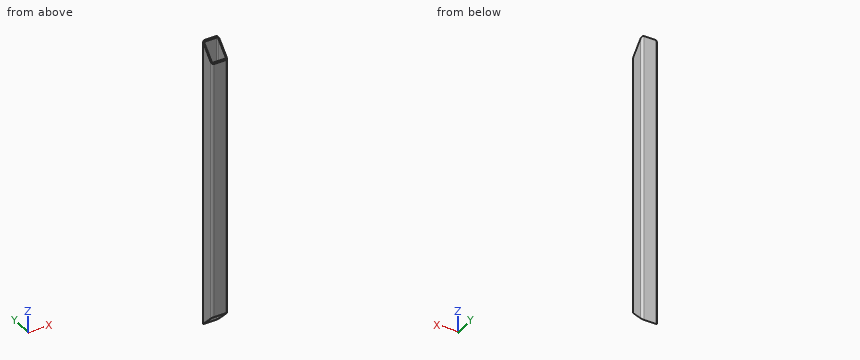
Autodesk Inventor part; units mm, degrees
ref_plane "Plano inicial" through (0, 0, 0) normal (0, 0, 1) x (1, 0, 0)
ref_plane "Plano final" through (0, 0, 550) normal (0, 0, 1) x (1, 0, 0)
ref_plane "Plano de trabalho6" through (15, 0, 0) normal (0, 0, -1) x (-1, 0, 0)
ref_plane "Plano inicial" through (0, 0, 0) normal (0, 0, 1) x (1, 0, 0)
ref_plane "Plano final" through (0, 0, 550) normal (0, 0, 1) x (1, 0, 0)
sketch "Esboço" plane through (0, 0, 0) normal (0, 0, 1) x (1, 0, 0)
  line L0 (-15, -11) -> (-15, 11)
  line L1 (-11, 15) -> (11, 15)
  line L2 (15, 11) -> (15, -11)
  line L3 (11, -15) -> (-11, -15)
  arc A0 (-15, -11) -> (-11, -15) centre (-11, -11) ccw
  arc A1 (15, 11) -> (11, 15) centre (11, 11) ccw
  arc A2 (-11, 15) -> (-15, 11) centre (-11, 11) ccw
  arc A3 (11, -15) -> (15, -11) centre (11, -11) ccw
  arc A4 (-11, 13) -> (-13, 11) centre (-11, 11) ccw
  line L4 (-11, 13) -> (11, 13)
  arc A5 (13, 11) -> (11, 13) centre (11, 11) ccw
  line L5 (13, 11) -> (13, -11)
  arc A6 (11, -13) -> (13, -11) centre (11, -11) ccw
  line L6 (11, -13) -> (-11, -13)
  arc A7 (-13, -11) -> (-11, -13) centre (-11, -11) ccw
  line L7 (-13, -11) -> (-13, 11)
  line L8 (0, 22.1598) -> (0, -22.1598) construction
  line L9 (-22.1598, 0) -> (22.1598, 0) construction
  dimension "d7" = 4
  dimension "d9" = 30
  dimension "d11" = 30
  dimension "d12" = 2
  dimension "d15" = 15
  dimension "d16" = 15
extrude "Corpo" add sketch "Esboço" along normal up to surface (550 mm away) from surface at 0
sketch "Sketch3" plane through (0, 0, 0) normal (0, 0, 1) x (1, 0, 0)
  line L0 (0, 0) -> (10, 0)
ref_plane "Work Plane3" through (0, 0, 0) normal (0, -1, 0) x (1, 0, 0)
sketch "Sketch4" plane through (0, 0, 0) normal (0, -1, 0) x (1, 0, 0)
  line L0 (-2, 0) -> (12, 0)
  line L1 (-2, 550) -> (12, 550)
  dimension "d18" = 550
ref_plane "Plano de trabalho6" through (15, 0, 0) normal (0, 0, -1) x (-1, 0, 0)
split "Dividir3" plane through (15, 0, 0) removes the side toward (0, 0, -1)
ref_plane "Plano de trabalho7" through (105, 0, 550) normal (0, 0, 1) x (1, 0, 0)
split "Dividir4" plane through (105, 0, 550) removes the side toward (0, 0, 1)
ref_plane "Plano de trabalho8" through (0, 15, 550) normal (0, -0.7071, 0.7071) x (1, 0, 0)
split "Dividir5" plane through (0, 15, 550) removes the side toward (0, -0.7071, 0.7071)
ref_plane "Plano de trabalho9" through (0, 15, -0.0001) normal (0, -0.7071, -0.7071) x (1, 0, 0)
split "Dividir6" plane through (0, 15, -0.0001) removes the side toward (0, -0.7071, -0.7071)
equation "\"d7\" = G_IR"
equation "\"d9\" = G_W"
equation "\"d11\" = G_H"
equation "\"d12\" = G_T"
equation "\"d15\" = 0.5 * d9"
equation "\"d16\" = 0.5 * d11"
equation "\"d3\" = G_L"
equation "\"G_W\" = 30"
equation "\"G_H\" = 30"
equation "\"G_T\" = 2"
equation "\"G_IR\" = 4"
equation "\"G_L\" = d18"
equation "\"G_OFFSET_START\" = 0"
equation "\"G_OFFSET_END\" = 0"
properties part number "ISO 10799-2 - 30x30x2 - 550" material "Aço, suave"
Read the model definition and answer for the solid it produces. Units are mm, in the model's axes. Give positions to 0.01 mm unless a question says otherwise; leave off trailing zeros. Write each loop counter-clockwise with the first axis right and the second up, starting at its lowest first coordinate (ties: lowest second). Pieces come first, ordered by that corner, then holes. Notation, with made-up numbers: (62, 10) - (80, 10) arc R18 ccw to (80, 44) - close; hole circle Ø8 at (6.25, -6.5). An arc over 180 degrees is marked (long way). Use CSV: the item, a comma, the result in double quotes. Start each with the question number.
Item 1: The part is cut by section C-C, the plane z = 427.5. Give the vertices of the cut face in (x, y), and give its area (3 significant figures).
Item 2: Consider line 1 (X direction, y = -9.75, z = 99.5); line 2 (X direction, y = -11.5, z = 267). Determine where each line is inside the solid, lowest interval first.
Item 3: The part is cut by section B-B, the plane y = -5.75. Give the vertices of the cut face in (x, z).
Taken from the geometry:
1,outline,"(-15, -11) arc R4 ccw to (-11, -15) - (11, -15) arc R4 ccw to (15, -11) - (15, 11) arc R4 ccw to (11, 15) - (-11, 15) arc R4 ccw to (-15, 11) - close; hole (-13, -11) arc R2 ccw to (-11, -13) - (11, -13) arc R2 ccw to (13, -11) - (13, 11) arc R2 ccw to (11, 13) - (-11, 13) arc R2 ccw to (-13, 11) - close"
1,area,"214 mm2"
2,line 1,"-15 to -13, 13 to 15"
2,line 2,"-14.97 to -12.94, 12.94 to 14.97"
3,outline,"(-15, 20.75) - (-13, 20.75) - (-13, 529.25) - (-15, 529.25) - close; (13, 20.75) - (15, 20.75) - (15, 529.25) - (13, 529.25) - close"
